Input: dimensioned drawing with shaded views. Units: mm. Origin: part minimum x, y, z. A direction names the side the tool comes from. Round coordinates to 2 decimals unless told otherwise and drop trailing zeros. Order: outer loops, then holes, each group sorted by start corner. A loop starts at its lowest first (then second) coordinate and runs counter-clockwise, first axis right, second up. Notation, with made-up numbers: (73.5, 75.5) - (96.5, 75.5) arc R27 cw to (96.5, 102.5) - close; hole circle Ø8 at (11, 9.5). An arc over 180 degrees is marked (long way). Return JSON: item names as keys, results as strings. Group by question number.
1) Contact query for flat-ended pins moving along their axis: P1, Ø2, axis at y = 24.5, z = 22.5, coming from the +X side; P2, Ø17, axis at x = 22.5, y = 16, coming from the +Z side; P3, Ø12, axis at x = 66.5, z = 9, coming from the +Y side; P4, Ø4, axis at x = 50, z = 29.5, coming from the +Y side. Output: stop coordinate, or through.
2) Section A-A, the plane x = 17.5. Return loops of the section in (y, z), plus the area to 3 significant figures.
3) Mould query, pull axis X, two halves, no side actions, for the marked faces 3, 4, 5 and 6. Classes: pulls with the +X half, pulls with the -X half, needs draft (parallel to the pull), parting line crosses it, or undercut.
4) Section C-C, the plane x = 26. Return loops of the section in (y, z).
5) Ray query, line 1 (X direction, y = 18, z = 7); line 2 (Y direction, x = 17.5, z = 3.8); line 3 (Z direction, x = 63.5, y = 33.5). Return the intervals inside material, ascending. Write a range as from..to.
6) Section B-B, the plane y = 4.5. Return loops of the section in (x, z) (1 decimal).
7) Access query for the marked faces 1 and 2. Directions: +Z, -Z, +X, -X, +Y, -Y. A direction counts if a zero-diameter tool reaches every point of the face in a straight line with its end or side. Return the directions, or none.
8) Section D-D, the plane z = 27.5. Give the number of separate pieces and of enclosed holes in the cut face.
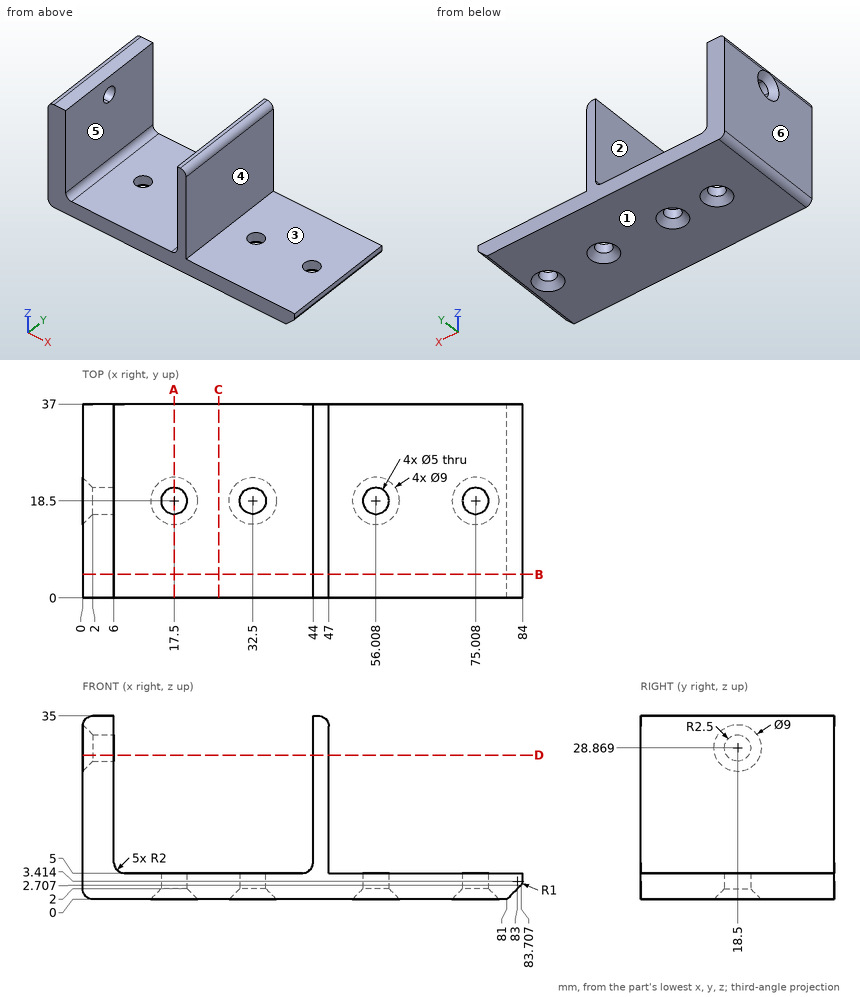
Geometry check:
{
 "1": {"P1": "x = 47", "P2": "z = 5", "P3": "y = 37", "P4": "through"},
 "2": {"outline": "(0, 0) - (14, 0) - (16, 2) - (16, 5) - (0, 5) - close; (21, 2) - (23, 0) - (37, 0) - (37, 5) - (21, 5) - close", "area": "156 mm2"},
 "3": {"face 3": "needs draft", "face 4": "pulls with the +X half", "face 5": "undercut", "face 6": "pulls with the -X half"},
 "4": {"outline": "(0, 0) - (37, 0) - (37, 5) - (0, 5) - close"},
 "5": {"line 1": "0..6, 44..47", "line 2": "0..16, 21..37", "line 3": "0..5"},
 "6": {"outline": "(0, 2) arc R2 ccw to (2, 0) - (81, 0) - (83.7, 2.7) arc R1 ccw to (84, 3.4) - (84, 5) - (47, 5) - (47, 33) arc R2 ccw to (45, 35) - (44, 35) - (44, 7) arc R2 cw to (42, 5) - (8, 5) arc R2 cw to (6, 7) - (6, 35) - (2, 35) arc R2 ccw to (0, 33) - close"},
 "7": {"face 1": "-Z, +X, -X, +Y, -Y", "face 2": "+Z, +Y, -Y"},
 "8": {"separate pieces": "3", "enclosed holes": "0"}
}
